Build history of the part. All positions in model axes, mm. Give positions to 0.01 mm unless a question says otherwise; leave off trailing zeros. Write each loop counter-clockwise with the first axis right and the second up, starting at its lowest first coordinate (ties: lowest second). Pieces come first, ordered by that corner, then holes. Notation, with made-up numbers: (-28.75, -34.5) -> (22.25, -34.5) arc R29 ccw to (22.25, -5.5) -> close; hole circle Ø9 at (7.25, -22). An arc over 180 degrees is marked (long way). Put each result on its own line as item: value.
from build123d import *

# Parameters (mm, degrees)
SKETCH1_W            = 90
SKETCH1_H            = 90
BOSS_EXTRUDE1_DEPTH  = 10
M6_CLEARANCE_HOLE2_D = 7
SKETCH3_R            = 6
CUT_EXTRUDE2_DEPTH   = 26
FILLET1_R            = 10


with BuildPart() as part:
    # Sketch1 → Boss-Extrude1 (new body)
    with BuildSketch(Plane(origin=(0, 0, 0), x_dir=(1, 0, 0), z_dir=(0, 1, 0))):
        Rectangle(SKETCH1_W, SKETCH1_H)
    extrude(amount=BOSS_EXTRUDE1_DEPTH)

    # M6 Clearance Hole2 (through all)
    with Locations(Plane(origin=(-35.5, 10, -35.5), x_dir=(0, 0, 1), z_dir=(0, 1, 0))):
        with Locations((0, 0), (0, 71), (71, 0), (71, 71)):
            Hole(M6_CLEARANCE_HOLE2_D / 2)

    # Sketch3 → Cut-Extrude2 (cut)
    with BuildSketch(Plane(origin=(0, 10, 0), x_dir=(1, 0, 0), z_dir=(0, 1, 0))):
        with Locations(Location((0, 25, 0), (0, 0, 270))):
            Circle(SKETCH3_R)
        with Locations(Location((-25, 0, 0), (0, 0, 270))):
            Circle(SKETCH3_R)
        with Locations(Location((0, -25, 0), (0, 0, 270))):
            Circle(SKETCH3_R)
        with Locations(Location((25, 0, 0), (0, 0, 270))):
            Circle(SKETCH3_R)
    extrude(amount=-CUT_EXTRUDE2_DEPTH, mode=Mode.SUBTRACT)

    # Fillet1
    fillet1_edges = [part.edges().sort_by_distance(p)[0] for p in [
        (45, 5, 45),
        (-45, 5, 45),
        (-45, 5, -45),
        (45, 5, -45),
    ]]
    fillet(fillet1_edges, radius=FILLET1_R)


solid = part.part
1) Pull direction Z, two halves, no side cores. Call faces 1 (the flat face through (0, 5, -45)), 2 (the cylindrical face through (37.865, 4.93, 38.08)), 3 (the flat face through (45, 5, 0)): released by +Z, released by -Z, zero draft, split by the parting line, or undercut.
Filled sheet:
face 1: released by -Z
face 2: undercut
face 3: zero draft
2) Slice it at B-B (y = 5.25). Give the number of separate pieces and of enclosed holes in the cut face, plus the area to 3 significant figures.
Filled sheet:
separate pieces: 1
enclosed holes: 8
area: 7,410 mm2
3) Wall check: L1, parallel to X at y = 4.5, z = 0; L2, parallel to X at y = 2.75, z = 35.5; L3, parallel to Z at x = 34, y = 8.5. Give the ranges that are in metal, low to high.
Filled sheet:
L1: -45 to -31, -19 to 19, 31 to 45
L2: -44.99 to -39, -32 to 32, 39 to 44.99
L3: -45 to -38.66, -32.34 to 32.34, 38.66 to 45
4) Slice it at C-C (z = 4). Write the cut outline in (x, y), plus the area to 3 significant figures.
Filled sheet:
outline: (-45, 0) -> (-29.47, 0) -> (-29.47, 10) -> (-45, 10) -> close; (-20.53, 0) -> (20.53, 0) -> (20.53, 10) -> (-20.53, 10) -> close; (29.47, 0) -> (45, 0) -> (45, 10) -> (29.47, 10) -> close
area: 721 mm2
5) Slice it at A-A (x = -25). Write the cut outline in (y, z).
Filled sheet:
outline: (0, -45) -> (10, -45) -> (10, -6) -> (0, -6) -> close; (0, 6) -> (10, 6) -> (10, 45) -> (0, 45) -> close
